Work out the finished part from the listing and answer in its coordinate system (mm). A direction names the side the tool comes from. Round coordinates to 2 decimals unless told otherwise and drop trailing zeros. Loops run counter-clockwise (first coordinate to the right, second up) from the corner with the lowest first, then second, coordinate; pieces in that order, holes last. Notation, with made-up numbers: (73, 85) -> (77, 85) arc R26 cw to (77, 119) -> close; hole circle Ø4 at (26, 85). An arc over 180 degrees is marked (long way). Use CSV: the item, a comma, the result in double quotes. Start each with the question number.
from build123d import *

# Parameters (mm, degrees)
SKETCH1_R           = 26.6192
BOSS_EXTRUDE1_DEPTH = 19.304
BOSS_EXTRUDE2_DEPTH = 15.7734
SKETCH3_R           = 12.7
CUT_EXTRUDE1_DEPTH  = 8.636
SKETCH4_R           = 5.55625
CUT_EXTRUDE2_DEPTH  = 47.003383041
FILLET1_R           = 1.27
FILLET2_R           = 1.27


with BuildPart() as part:
    # Sketch1 → Boss-Extrude1 (new body)
    with BuildSketch(Plane(origin=(0, 0, 0), x_dir=(1, 0, 0), z_dir=(0, 1, 0))):
        with Locations(Location((0, 0, 0), (0, 0, 270))):
            Circle(SKETCH1_R)
    extrude(amount=BOSS_EXTRUDE1_DEPTH)

    # Sketch2 → Boss-Extrude2 (add)
    with BuildSketch(Plane(origin=(0, 19.304, 0), x_dir=(1, 0, 0), z_dir=(0, 1, 0))):
        with BuildLine():
            Line((-6.6675, 14.546767605), (-6.6675, 24.892))
            Line((-6.6675, 24.892), (6.6675, 24.892))
            Line((6.6675, 24.892), (6.6675, 14.546767605))
            ThreePointArc((6.6675, 14.546767605), (11.315122713, 11.315122713), (14.546767605, 6.6675))
            Line((14.546767605, 6.6675), (24.892, 6.6675))
            Line((24.892, 6.6675), (24.892, -6.6675))
            Line((24.892, -6.6675), (14.546767605, -6.6675))
            ThreePointArc((14.546767605, -6.6675), (11.315122713, -11.315122713), (6.6675, -14.546767605))
            Line((6.6675, -14.546767605), (6.6675, -24.892))
            Line((6.6675, -24.892), (-6.6675, -24.892))
            Line((-6.6675, -24.892), (-6.6675, -14.546767605))
            ThreePointArc((-6.6675, -14.546767605), (-11.315122713, -11.315122713), (-14.546767605, -6.6675))
            Line((-14.546767605, -6.6675), (-24.892, -6.6675))
            Line((-24.892, -6.6675), (-24.892, 6.6675))
            Line((-24.892, 6.6675), (-14.546767605, 6.6675))
            ThreePointArc((-14.546767605, 6.6675), (-11.315122713, 11.315122713), (-6.6675, 14.546767605))
        make_face()
    extrude(amount=BOSS_EXTRUDE2_DEPTH)

    # Sketch3 → Cut-Extrude1 (cut)
    with BuildSketch(Plane(origin=(0, 35.0774, 0), x_dir=(1, 0, 0), z_dir=(0, 1, 0))):
        with Locations(Location((0, 0, 0), (0, 0, 270))):
            Circle(SKETCH3_R)
    extrude(amount=-CUT_EXTRUDE1_DEPTH, mode=Mode.SUBTRACT)

    # Sketch4 → Cut-Extrude2 (cut, through all)
    with BuildSketch(Plane(origin=(0, 26.4414, 0), x_dir=(1, 0, 0), z_dir=(0, 1, 0))):
        with Locations(Location((0, 0, 0), (0, 0, 270))):
            Circle(SKETCH4_R)
    extrude(amount=-CUT_EXTRUDE2_DEPTH, mode=Mode.SUBTRACT)

    # Fillet1
    fillet1_edges = [part.edges().sort_by_distance(p)[0] for p in [
        (-11.315122713, 35.0774, -11.315122713),
        (-19.719383802, 35.0774, -6.6675),
        (-24.892, 35.0774, 0),
        (-19.719383802, 35.0774, 6.6675),
        (-11.315122713, 35.0774, 11.315122713),
        (-6.6675, 35.0774, 19.719383802),
        (0, 35.0774, 24.892),
        (6.6675, 35.0774, 19.719383802),
        (11.315122713, 35.0774, 11.315122713),
        (19.719383802, 35.0774, 6.6675),
        (24.892, 35.0774, 0),
        (19.719383802, 35.0774, -6.6675),
        (11.315122713, 35.0774, -11.315122713),
        (6.6675, 35.0774, -19.719383802),
        (0, 35.0774, -24.892),
        (-6.6675, 35.0774, -19.719383802),
    ]]
    fillet(fillet1_edges, radius=FILLET1_R)

    # Fillet2
    # the kernel refuses this fillet: 1.27 mm, written as the material it takes off along each edge
    with BuildSketch(Plane(origin=(5.3975, 33.8074, -23.622), x_dir=(0, 0, -1), z_dir=(1, 0, 0))) as fillet2_piece_1_section:
        Polygon((0, 0), (FILLET2_R, 0), (FILLET2_R, FILLET2_R), (0, FILLET2_R), align=None)
    fillet2_piece_1 = extrude(amount=FILLET2_R, mode=Mode.PRIVATE)
    fillet2_piece_1 = fillet2_piece_1 - Plane(origin=(5.3975, 33.8074, -23.622), x_dir=(0, -0.7071067811865475, 0.7071067811865475), z_dir=(1, 0, 0)) * Sphere(FILLET2_R, mode=Mode.PRIVATE)
    add(fillet2_piece_1, mode=Mode.SUBTRACT)
    with BuildSketch(Plane(origin=(23.622, 33.8074, -5.3975), x_dir=(0, 0, -1), z_dir=(1, 0, 0))) as fillet2_piece_2_section:
        Polygon((0, 0), (FILLET2_R, 0), (FILLET2_R, FILLET2_R), (0, FILLET2_R), align=None)
    fillet2_piece_2 = extrude(amount=FILLET2_R, mode=Mode.PRIVATE)
    fillet2_piece_2 = fillet2_piece_2 - Plane(origin=(23.622, 33.8074, -5.3975), x_dir=(0, -0.7071067811865475, 0.7071067811865475), z_dir=(1, 0, 0)) * Sphere(FILLET2_R, mode=Mode.PRIVATE)
    add(fillet2_piece_2, mode=Mode.SUBTRACT)
    with BuildSketch(Plane(origin=(-5.3975, 33.8074, -23.622), x_dir=(0, 0, -1), z_dir=(-1, 0, 0))) as fillet2_piece_3_section:
        Polygon((0, 0), (FILLET2_R, 0), (FILLET2_R, -FILLET2_R), (0, -FILLET2_R), align=None)
    fillet2_piece_3 = extrude(amount=FILLET2_R, mode=Mode.PRIVATE)
    fillet2_piece_3 = fillet2_piece_3 - Plane(origin=(-5.3975, 33.8074, -23.622), x_dir=(0, -0.7071067811865475, 0.7071067811865475), z_dir=(-1, 0, 0)) * Sphere(FILLET2_R, mode=Mode.PRIVATE)
    add(fillet2_piece_3, mode=Mode.SUBTRACT)
    with BuildSketch(Plane(origin=(23.622, 33.8074, 5.3975), x_dir=(1, 0, 0), z_dir=(0, 0, 1))) as fillet2_piece_4_section:
        Polygon((0, 0), (FILLET2_R, 0), (FILLET2_R, FILLET2_R), (0, FILLET2_R), align=None)
    fillet2_piece_4 = extrude(amount=FILLET2_R, mode=Mode.PRIVATE)
    fillet2_piece_4 = fillet2_piece_4 - Plane(origin=(23.622, 33.8074, 5.3975), x_dir=(-0.7071067811865475, -0.7071067811865475, 0), z_dir=(0, 0, 1)) * Sphere(FILLET2_R, mode=Mode.PRIVATE)
    add(fillet2_piece_4, mode=Mode.SUBTRACT)
    with BuildSketch(Plane(origin=(-23.622, 33.8074, -5.3975), x_dir=(-1, 0, 0), z_dir=(0, 0, -1))) as fillet2_piece_5_section:
        Polygon((0, 0), (FILLET2_R, 0), (FILLET2_R, FILLET2_R), (0, FILLET2_R), align=None)
    fillet2_piece_5 = extrude(amount=FILLET2_R, mode=Mode.PRIVATE)
    fillet2_piece_5 = fillet2_piece_5 - Plane(origin=(-23.622, 33.8074, -5.3975), x_dir=(0.7071067811865475, -0.7071067811865475, 0), z_dir=(0, 0, -1)) * Sphere(FILLET2_R, mode=Mode.PRIVATE)
    add(fillet2_piece_5, mode=Mode.SUBTRACT)
    with BuildSketch(Plane(origin=(5.3975, 33.8074, 23.622), x_dir=(1, 0, 0), z_dir=(0, 0, 1))) as fillet2_piece_6_section:
        Polygon((0, 0), (FILLET2_R, 0), (FILLET2_R, FILLET2_R), (0, FILLET2_R), align=None)
    fillet2_piece_6 = extrude(amount=FILLET2_R, mode=Mode.PRIVATE)
    fillet2_piece_6 = fillet2_piece_6 - Plane(origin=(5.3975, 33.8074, 23.622), x_dir=(-0.7071067811865475, -0.7071067811865475, 0), z_dir=(0, 0, 1)) * Sphere(FILLET2_R, mode=Mode.PRIVATE)
    add(fillet2_piece_6, mode=Mode.SUBTRACT)
    with BuildSketch(Plane(origin=(-23.622, 33.8074, 5.3975), x_dir=(0, 0, 1), z_dir=(-1, 0, 0))) as fillet2_piece_7_section:
        Polygon((0, 0), (FILLET2_R, 0), (FILLET2_R, FILLET2_R), (0, FILLET2_R), align=None)
    fillet2_piece_7 = extrude(amount=FILLET2_R, mode=Mode.PRIVATE)
    fillet2_piece_7 = fillet2_piece_7 - Plane(origin=(-23.622, 33.8074, 5.3975), x_dir=(0, -0.7071067811865475, -0.7071067811865475), z_dir=(-1, 0, 0)) * Sphere(FILLET2_R, mode=Mode.PRIVATE)
    add(fillet2_piece_7, mode=Mode.SUBTRACT)
    with BuildSketch(Plane(origin=(-5.3975, 33.8074, 23.622), x_dir=(0, 0, 1), z_dir=(-1, 0, 0))) as fillet2_piece_8_section:
        Polygon((0, 0), (FILLET2_R, 0), (FILLET2_R, FILLET2_R), (0, FILLET2_R), align=None)
    fillet2_piece_8 = extrude(amount=FILLET2_R, mode=Mode.PRIVATE)
    fillet2_piece_8 = fillet2_piece_8 - Plane(origin=(-5.3975, 33.8074, 23.622), x_dir=(0, -0.7071067811865475, -0.7071067811865475), z_dir=(-1, 0, 0)) * Sphere(FILLET2_R, mode=Mode.PRIVATE)
    add(fillet2_piece_8, mode=Mode.SUBTRACT)
    with BuildSketch(Plane(origin=(-6.6675, 19.304, 24.892), x_dir=(0, 0, -1), z_dir=(0, 1, 0)), Plane(origin=(6.6675, 19.304, 24.892), x_dir=(-1, 0, 0), z_dir=(0, 1, 0)), Plane(origin=(24.892, 19.304, 6.6675), x_dir=(-1, 0, 0), z_dir=(0, 1, 0)), Plane(origin=(24.892, 19.304, -6.6675), x_dir=(0, 0, 1), z_dir=(0, 1, 0)), Plane(origin=(6.6675, 19.304, -24.892), x_dir=(0, 0, 1), z_dir=(0, 1, 0)), Plane(origin=(-24.892, 19.304, -6.6675), x_dir=(1, 0, 0), z_dir=(0, 1, 0)), Plane(origin=(-24.892, 19.304, 6.6675), x_dir=(0, 0, -1), z_dir=(0, 1, 0))) as fillet2_piece_9:
        with BuildLine():
            CenterArc((FILLET2_R, -FILLET2_R), FILLET2_R, 90, 90)
            Line((0, -FILLET2_R), (0, 0))
            Line((0, 0), (FILLET2_R, 0))
        make_face()
    extrude(amount=14.5034, mode=Mode.SUBTRACT)
    with BuildSketch(Plane(origin=(-6.6675, 19.304, -24.892), x_dir=(0, 0, 1), z_dir=(0, 1, 0))) as fillet2_piece_10:
        with BuildLine():
            CenterArc((FILLET2_R, FILLET2_R), FILLET2_R, 180, 90)
            Line((0, FILLET2_R), (0, 0))
            Line((0, 0), (FILLET2_R, 0))
        make_face()
    extrude(amount=14.5034, mode=Mode.SUBTRACT)


solid = part.part
Q1. Section A-A, the plane x = 0 is taken. Write down the section's boundary in (y, z).
Q2. Section C-C, the plane y = 32 is taken. Write down the section's boundary in (x, z).
Q3. Section D-D, the plane z = -16.5 is taken. Write down the section's boundary in (x, y), and give its area (3 significant figures).
Q4. Which of the six approach directions +Z, -Z, +X, -X, +Y, -Y give full straight-line access (tool end or side, diameter ignored) to faces 4 (the flat face through (24.892, 26, 0)), 5 (the cylindrical face through (24.53, 26.454, -6.286)), 6 (the cylindrical face through (-6.3, 34.7, 18.6))?
Q5. Each of these flat-tipped pins is pushed along its axis until it touches: pin 1 (8 mm diameter, centred on y = 18, z = -14, fed in from +X); pin 2 (10 mm diameter, centred on x = 17, y = 27, fed in from +Z); pin 3 (1 mm diameter, centred on y = 20.5, z = -5.5, fed in from +X); pin 4 (20.5 mm diameter, centred on x = 2, z = 4.5, fed in from +Y). Where does it stop, or does it pass through?
Q6. Straight lines are drawn through the part: line 1 (Y direction, x = -5.5, z = 8.5); line 2 (X direction, y = 20.5, z = 19.5); line 3 (Y direction, x = 15, z = 16). For each, find the intervals that lie inside material, in ascending order. Write a range as from..to.
Q7. For a pull along X with two mould halves and no side action, classify faces 1 (the flat face through (-3, 26.441, 5)), 2 (the flat face through (0, 26, 24.892)), 3 (the flat face through (6.668, 26, -19)) as pulls with the +X half, pulls with the -X half, needs draft (parallel to the pull), parting line crosses it, or undercut.
Q8. Section B-B, the plane z = 0 is taken. Write down the section's boundary in (x, y), and give its area (3 significant figures).
Report:
1,outline,"(0, -26.62) -> (19.3, -26.62) -> (19.3, -24.89) -> (33.81, -24.89) arc R1.27 ccw to (35.08, -23.62) -> (35.08, -12.7) -> (26.44, -12.7) -> (26.44, -5.56) -> (0, -5.56) -> close; (0, 5.56) -> (26.44, 5.56) -> (26.44, 12.7) -> (35.08, 12.7) -> (35.08, 23.62) arc R1.27 ccw to (33.81, 24.89) -> (19.3, 24.89) -> (19.3, 26.62) -> (0, 26.62) -> close"
2,outline,"(-24.89, -5.4) arc R1.27 ccw to (-23.62, -6.67) -> (-14.55, -6.67) arc R16 ccw to (-6.67, -14.55) -> (-6.67, -23.62) arc R1.27 ccw to (-5.4, -24.89) -> (5.4, -24.89) arc R1.27 ccw to (6.67, -23.62) -> (6.67, -14.55) arc R16 ccw to (14.55, -6.67) -> (23.62, -6.67) arc R1.27 ccw to (24.89, -5.4) -> (24.89, 5.4) arc R1.27 ccw to (23.62, 6.67) -> (14.55, 6.67) arc R16 ccw to (6.67, 14.55) -> (6.67, 23.62) arc R1.27 ccw to (5.4, 24.89) -> (-5.4, 24.89) arc R1.27 ccw to (-6.67, 23.62) -> (-6.67, 14.55) arc R16 ccw to (-14.55, 6.67) -> (-23.62, 6.67) arc R1.27 ccw to (-24.89, 5.4) -> close; hole circle Ø25.4 at (0, 0)"
3,outline,"(-20.89, 0) -> (20.89, 0) -> (20.89, 19.3) -> (6.67, 19.3) -> (6.67, 33.81) arc R1.27 ccw to (5.4, 35.08) -> (-5.4, 35.08) arc R1.27 ccw to (-6.67, 33.81) -> (-6.67, 19.3) -> (-20.89, 19.3) -> close"
3,area,"1,020 mm²"
4,face 4,"+Z, -Z, +X, +Y"
4,face 5,"-Z, +X, +Y"
4,face 6,"+Z, -X, +Y"
5,pin 1,"stops at x = 24.67"
5,pin 2,"stops at z = 10.59"
5,pin 3,"stops at x = 24.89"
5,pin 4,"stops at y = 35.08"
6,line 1,"y = 0..26.44"
6,line 2,"x = -6.67..6.67"
6,line 3,"y = 0..19.3"
7,face 1,"undercut"
7,face 2,"needs draft"
7,face 3,"pulls with the +X half"
8,outline,"(-26.62, 0) -> (-5.56, 0) -> (-5.56, 26.44) -> (-12.7, 26.44) -> (-12.7, 35.08) -> (-23.62, 35.08) arc R1.27 ccw to (-24.89, 33.81) -> (-24.89, 19.3) -> (-26.62, 19.3) -> close; (5.56, 0) -> (26.62, 0) -> (26.62, 19.3) -> (24.89, 19.3) -> (24.89, 33.81) arc R1.27 ccw to (23.62, 35.08) -> (12.7, 35.08) -> (12.7, 26.44) -> (5.56, 26.44) -> close"
8,area,"1,300 mm²"
